The drawing under review shows one solid part. Ordinate dimensions are in mm from its lowest x, y, z. Give positions to 0.01 mm unless a question says otherwise; leave off trailing zeros. Loops run counter-clockwise (first coordinate to the right, second up) from the corner with the lowest first, then second, coordinate; pieces in that order, holes last. Notation, with made-up numbers: M 49,-7 L 62,-7 A21 cw 62,29 Z; hole C -26,54 d9. An arc over 180 degrees is marked long. One line per item, written item: value. Start each with the question number.
Q1. To check wall thickness, follow line 1 along Y through (x, z) = (7.5, 0.75); line 2 along X through (y, z) = (7.25, 0.8); line 3 along Y through (x, z) = (11.5, 2.1) (1 decimal). State the ranges of each line that lie inside material, in increasing order. Write a range as from..to.
Q2. We need section A-A on x = 8.75. Write out the cut boundary in (y, z), plus the area to 3 significant figures.
Q3. Mouldability with a two-part tool opening along X and no side actions: class the marked faces 1, 2 and 3 as released by +X, released by -X, zero draft, split by the parting line, or undercut.
Q4. For pin 1 (1.5 mm diameter, centred on x = 12, z = 4, fed in from -Y); pin 2 (3 mm diameter, centred on y = 9.5, z = 1, fed in from -X); pin 3 (1.5 mm diameter, centred on y = 1.5, z = 1.5, fed in from +X); pin 4 (3 mm diameter, centred on x = 8.39, y = 7.9, fed in from +Z), all flat-tipped, find the tip position at first contact; note any pin that passes through.
Q5. We need section B-B on y = 7.9. Write out the cut boundary in (x, z), plus the area to 3 significant figures.
Q6. We need section C-C on y = 12. Write out the cut boundary in (x, z), plus the area to 3 significant figures.
Q7. We need section D-D on z = 4.1. Write out the cut boundary in (x, y), plus the area to 3 significant figures.
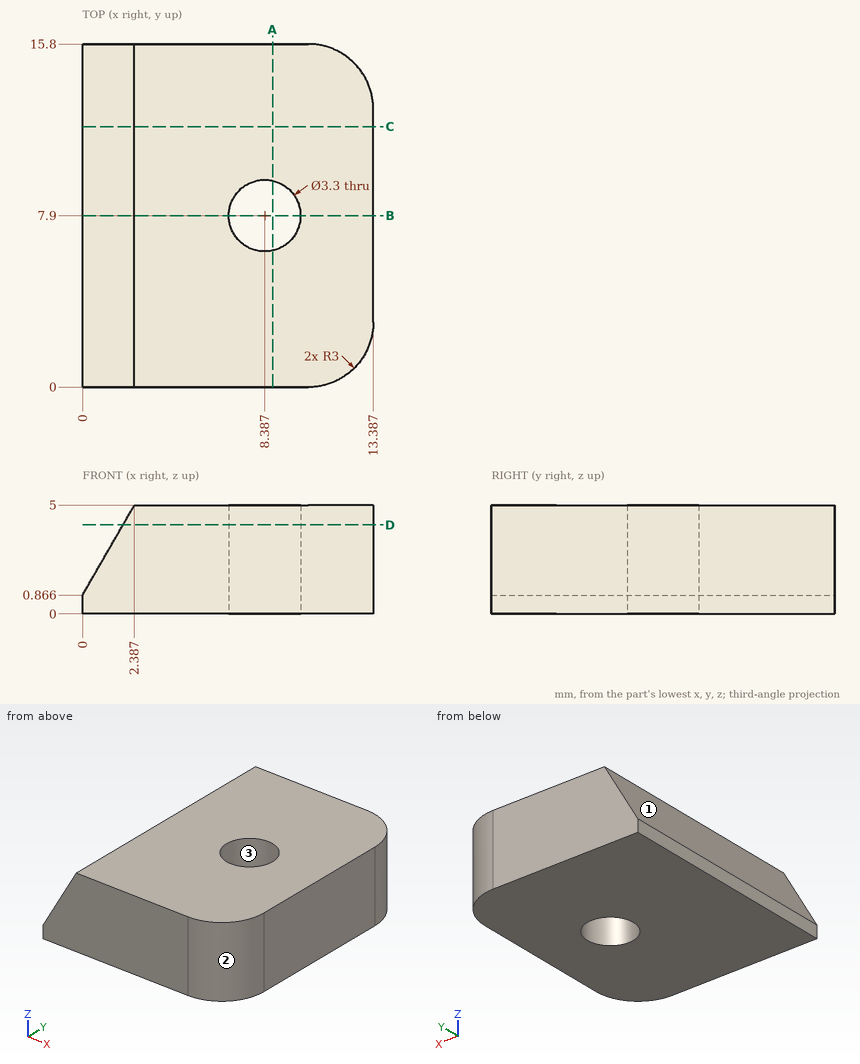
Solved:
1. line 1: 0..6.51, 9.29..15.8
1. line 2: 0..6.87, 9.9..13.39
1. line 3: 0.2..15.6
2. outline: M 0,0 L 6.29,0 L 6.29,5 L 0,5 Z; M 9.51,0 L 15.8,0 L 15.8,5 L 9.51,5 Z
2. area: 62.9 mm2
3. face 1: released by -X
3. face 2: released by +X
3. face 3: undercut
4. pin 1: y = 0.13
4. pin 2: x = 0
4. pin 3: x = 13.29
4. pin 4: through
5. outline: M 0,0 L 6.74,0 L 6.74,5 L 2.39,5 L 0,0.87 Z; M 10.04,0 L 13.39,0 L 13.39,5 L 10.04,5 Z
5. area: 45.5 mm2
6. outline: M 0,0 L 13.39,0 L 13.39,5 L 2.39,5 L 0,0.87 Z
6. area: 62.0 mm2
7. outline: M 1.87,0 L 10.39,0 A3 ccw 13.39,3 L 13.39,12.8 A3 ccw 10.39,15.8 L 1.87,15.8 Z; hole C 8.39,7.9 d3.3
7. area: 170 mm2
